Here's how the part is built. I have some questions about the finished solid (model axes, mm). Round coordinates to 2 decimals unless told otherwise and drop trailing zeros. Order: outer loops, then holes, each group sorted by start corner. A loop starts at its lowest first (then second) coordinate and runs counter-clockwise, first axis right, second up. Notation, with made-up numbers: M 12.25,25.5 L 69.25,25.5 A14 ccw 69.25,36.5 Z; hole C -19.75,31.5 d5. An arc over 180 degrees is marked long. Write item = value, one per line. Start each with the question number.
Item 1: I want a section at B-B, the plane x = -25.9. List the corners of the cut face in (y, z) for me (3 decimals), plus the area to 3 significant figures.
Item 2: Please list where these lines run through material, in increasing order: L1, parallel to Y at x = 31.75, z = 5.5; L2, parallel to Y at x = 25.9, z = 2.5; L3, parallel to X at y = 51, z = 6.5.
Item 3: I want a section at A-A, the plane y = -19.15. List the corners of the cut face in (x, z) for me (3 decimals), plus the area to 3 significant figures.
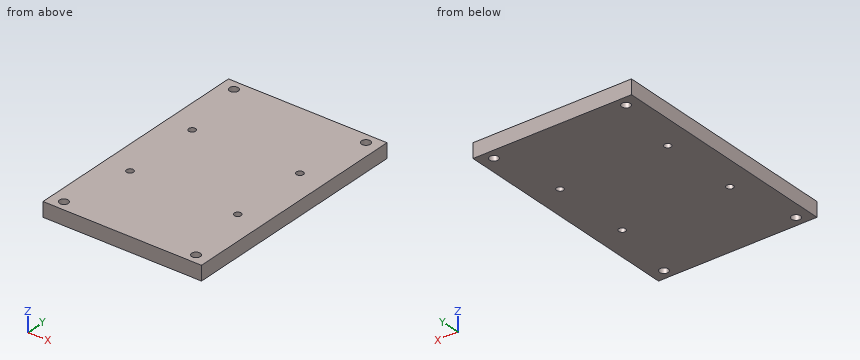
```python
from build123d import *

# Parameters (mm, degrees)
F0_W     = 76.2
F0_H     = 114.3
F1_DEPTH = 6.985
F3_D     = 4.2
F6_D     = 3.3
F6_DEPTH = 12
F6_TIP   = 0.9914200214


# Not quite as in the source:
# - a pattern or mirror of a feature is missing from the dataset's text; its kind, count and spacing are read off the source's solid
# - a feature names something its author has since deleted; it is built from what else it names


with BuildPart() as f1:
    # F0 (on Top) → F1 (new body)
    with BuildSketch(Plane.XY):
        Rectangle(F0_W, F0_H)
    extrude(amount=F1_DEPTH)

    # F3 (through all)
    with Locations(Plane.XY.offset(6.985)):
        with Locations((-31.75, 52.3875), (31.75, 52.3875), (31.75, -52.3875), (-31.75, -52.3875)):
            Hole(F3_D / 2)

    # F6
    with Locations(Plane.XY.offset(6.985)):
        with Locations((-25.9, -19.15), (25.9, -19.15)):
            f6 = Hole(F6_D / 2, depth=F6_DEPTH)
            with Locations((0, 0, -(F6_DEPTH + F6_TIP / 2))):  # 118° drill point
                Cone(0, F6_D / 2, F6_TIP, mode=Mode.SUBTRACT)

    # F6_copies: F6 across plane
    add(f6.mirror(Plane.ZX), mode=Mode.SUBTRACT)


solid = f1.part
```
Filled in:
q1.outline = M -57.15,0 L -20.8,0 L -20.8,6.985 L -57.15,6.985 Z; M -17.5,0 L 17.5,0 L 17.5,6.985 L -17.5,6.985 Z; M 20.8,0 L 57.15,0 L 57.15,6.985 L 20.8,6.985 Z
q1.area = 752 mm^2
q2.L1 = -57.15 to -54.49, -50.29 to 50.29, 54.49 to 57.15
q2.L2 = -57.15 to -20.8, -17.5 to 17.5, 20.8 to 57.15
q2.L3 = -38.1 to -33.33, -30.17 to 30.17, 33.33 to 38.1
q3.outline = M -38.1,0 L -27.55,0 L -27.55,6.985 L -38.1,6.985 Z; M -24.25,0 L 24.25,0 L 24.25,6.985 L -24.25,6.985 Z; M 27.55,0 L 38.1,0 L 38.1,6.985 L 27.55,6.985 Z
q3.area = 486 mm^2
